The listing builds one solid part. Answer for the finished solid, in the listing's coordinates (mm). Face numbers are marked on the shaded views. A direction names the side the tool comes from. Give positions to 0.01 mm unless a question says otherwise; leave off trailing zeros. Order: outer loops, then holes, each group sorted by start corner. A loop starts at its lowest first (then second) coordinate and runs counter-clockwise, first axis right, second up. Notation, with made-up numbers: (-28, 14) - (-10, 14) arc R18 cw to (-10, 44) - close; hole circle Ø5 at (-4.75, -37.5). An arc over 180 degrees is marked (long way). Answer in a Markdown table with one row per item.
from build123d import *

# Parameters (mm, degrees)
FILLET1_R           = 1.5
CHAMFER1_SIZE       = 0.5
BOSS_EXTRUDE1_DEPTH = 14.5


with BuildPart() as part:
    # Sketch1 → Revolve1 (revolve)
    with BuildSketch(Plane(origin=(0, 0, 0), x_dir=(1, 0, 0), z_dir=(0, 1, 0))):
        with BuildLine():
            Line((0, 0), (0, 100.5))
            Line((0, 100.5), (9.75, 100.5))
            Line((9.75, 100.5), (9.75, 90.5))
            ThreePointArc((9.75, 90.5), (8.441852455, 89.958147545), (7.9, 88.65))
            ThreePointArc((7.9, 88.65), (10.694495807, 84.667609495), (12.5, 80.15))
            Line((12.5, 80.15), (12.5, 69.15))
            ThreePointArc((12.5, 69.15), (11.395638202, 66.053286337), (9.822505168, 63.166332415))
            ThreePointArc((9.822505168, 63.166332415), (8.435454872, 60.164407444), (7.96, 56.89188476))
            Line((7.96, 56.89188476), (7.96, 44.9))
            Line((7.96, 44.9), (9.2, 44.9))
            Line((9.2, 44.9), (9.2, 16.5))
            Line((9.2, 16.5), (8, 16.5))
            Line((8, 16.5), (8, 11.5))
            ThreePointArc((8, 11.5), (6.585786438, 10.914213562), (6, 9.5))
            Line((6, 9.5), (6, 0))
            Line((6, 0), (0, 0))
        make_face()
    revolve(axis=Axis((0, 0, 0), (0, 0, -1)))

    # Fillet1
    fillet1_edges = [part.edges().sort_by_distance(p)[0] for p in [
        (-9.75, 0, -100.5),
    ]]
    fillet(fillet1_edges, radius=FILLET1_R)

    # Chamfer1
    chamfer1_edges = [part.edges().sort_by_distance(p)[0] for p in [
        (-6, 0, 0),
    ]]
    chamfer(chamfer1_edges, length=CHAMFER1_SIZE)

    # Sketch2 → Boss-Extrude1 (add)
    with BuildSketch(Plane.XY):
        Polygon((1.732050808, 3), (-1.732050808, 3), (-3.464101615, 0), (-1.732050808, -3), (1.732050808, -3), (3.464101615, 0), align=None)
    extrude(amount=BOSS_EXTRUDE1_DEPTH)

    # Sketch3 → Cut-Revolve1 (revolve, cut)
    with BuildSketch(Plane(origin=(0, 0, 0), x_dir=(1, 0, 0), z_dir=(0, 1, 0))):
        with BuildLine():
            Line((3, -14.5), (3, -4.5))
            ThreePointArc((3, -4.5), (3.1186767, -3.714921929), (3.464101615, -3))
            Line((3.464101615, -3), (3.464101615, -14.5))
            Line((3.464101615, -14.5), (3, -14.5))
        make_face()
    revolve(axis=Axis((0, 0, 0), (0, 0, 1)), mode=Mode.SUBTRACT)


solid = part.part
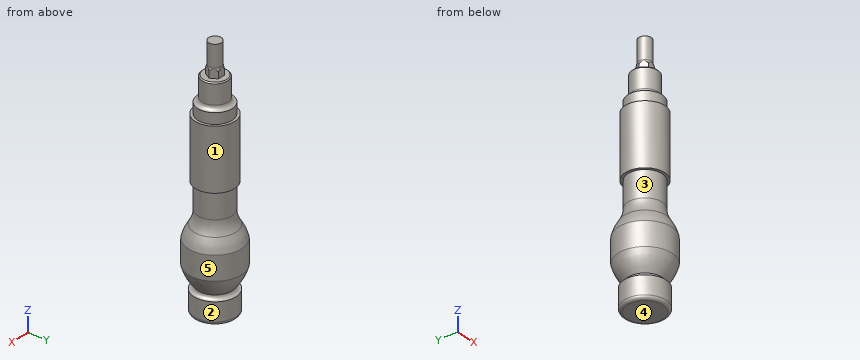
Item 1: Which of the six approach directions +Z, -Z, +X, -X, +Y, -Y give full straight-line access (tool end or side, diameter ignored) to the marked faces 1 and 2?
Answer block:
| item | result |
|---|---|
| face 1 | +Z |
| face 2 | -Z |
Item 2: Consider line 1 (Z direction, x = -5.75, y = 6.75); line 2 (Z direction, x = -2, y = -9.25); line 3 (Y direction, x = -0.5, z = -79). Determine where each line is inside the solid, lowest interval first.
Answer block:
| item | result |
|---|---|
| line 1 | -100.37 to -90.28, -87.48 to -61.37, -44.9 to -16.5 |
| line 2 | -99.88 to -90.48, -86.67 to -62.58 |
| line 3 | -12.49 to 12.49 |
Item 3: Determine the mould class of the marked faces 3, 4 and 5 for opening direction Z: pulls with the +Z half, pulls with the -Z half, needs draft (parallel to the pull), parting line crosses it, or undercut.
Answer block:
| item | result |
|---|---|
| face 3 | undercut |
| face 4 | pulls with the -Z half |
| face 5 | needs draft |
Item 4: Find section B-B on z = 6. Write down the section's boundary in (x, y), then the cut area to 3 significant figures.
Answer block:
| item | result |
|---|---|
| outline | circle Ø6 at (0, 0) |
| area | 28.3 mm² |
Item 5: Each of these flat-tipped pins is pushed along its axis until it touches: P1, Ø4, axis at y = -4.5, z = -50, coming from the +X side; P2, Ø6, axis at x = -9.5, z = -74, coming from the +Y side; P3, Ø1, axis at x = 0, z = 2.5, coming from the -Y side. Where does it stop, or does it pass through?
Answer block:
| item | result |
|---|---|
| P1 | x = 7.56 |
| P2 | y = 10.68 |
| P3 | y = -3 |
Item 6: Find section A-A on z = -33. Write down the section's boundary in (x, y), then the cut area to 3 significant figures.
Answer block:
| item | result |
|---|---|
| outline | circle Ø18.4 at (0, 0) |
| area | 266 mm² |
